Answer from the drawing. Dimensions are ordinates in mm from the lowest x, y and z of the part. A direction names the side the tool comes from. Give positions to 0.01 mm unless a question says otherwise; leave off trailing zeros. Write each loop counter-clockwise with the first axis right and the second up, starting at its lowest first coordinate (ties: lowest second). Pieces come first, ordered by that corner, then holes.
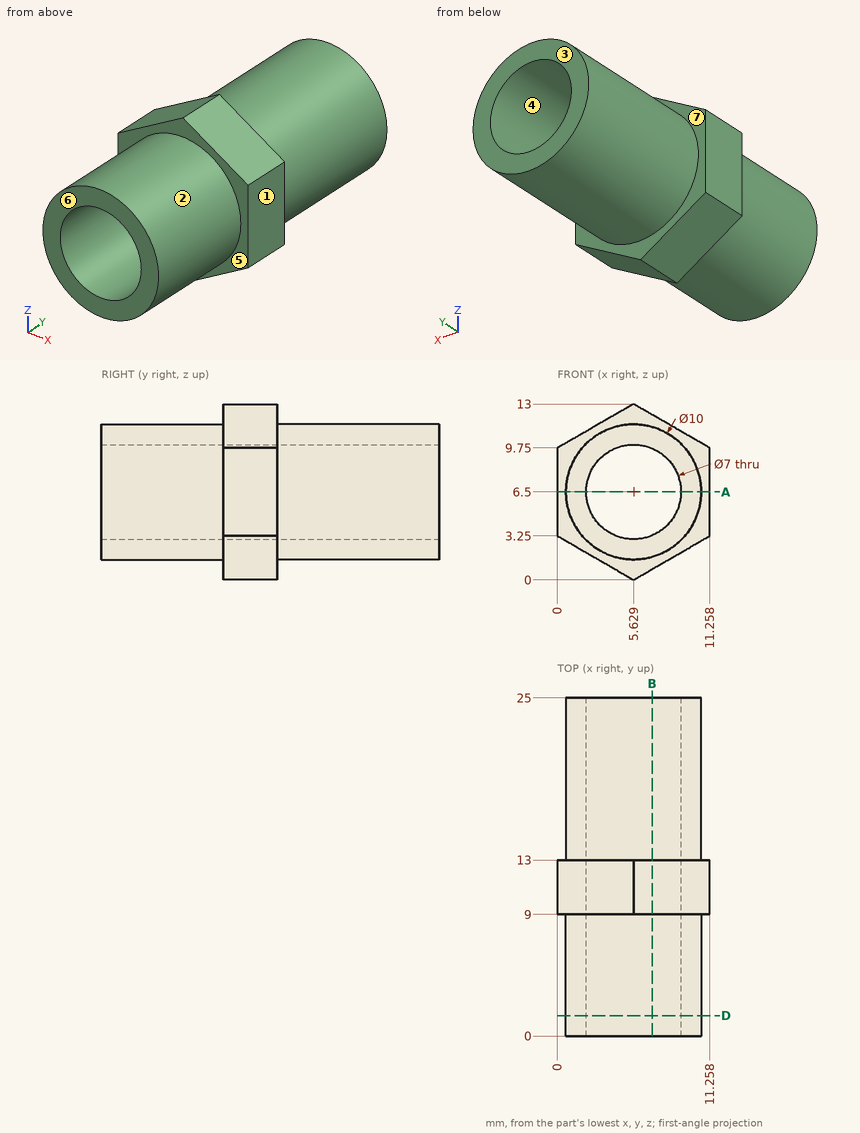
Item 1: A cutting plane is placed at D-D, the plane y = 1.5. Give the vertices of the cut face in (x, z).
Conclusion:
outline: circle Ø10 at (5.63, 6.5); hole circle Ø7 at (5.63, 6.5)
Item 2: Consider probe 1 along Z at (x, y) = (8, 12.5) (1 decimal); probe 2 along X at (y, z) = (18, 3.5) (1 decimal); probe 3 along Z at (x, y) = (4.5, 8.75). Determine where each line is inside the solid, lowest interval first.
Conclusion:
probe 1: z = 1.4 to 3.9, 9.1 to 11.6
probe 2: x = 1.6 to 3.8, 7.4 to 9.6
probe 3: z = 1.63 to 3.19, 9.81 to 11.37
Item 3: A cutting plane is placed at B-B, the plane x = 7. Give the vertices of the cut face in (y, z).
Conclusion:
outline: (0, 1.69) - (9, 1.69) - (9, 0.79) - (13, 0.79) - (13, 1.69) - (25, 1.69) - (25, 3.28) - (0, 3.28) - close; (0, 9.72) - (25, 9.72) - (25, 11.31) - (13, 11.31) - (13, 12.21) - (9, 12.21) - (9, 11.31) - (0, 11.31) - close
Item 4: A cutting plane is placed at A-A, the plane z = 6.5. Give the vertices of the cut face in (x, y).
Conclusion:
outline: (0, 9) - (0.63, 9) - (0.63, 0) - (2.13, 0) - (2.13, 25) - (0.63, 25) - (0.63, 13) - (0, 13) - close; (9.13, 0) - (10.63, 0) - (10.63, 9) - (11.26, 9) - (11.26, 13) - (10.63, 13) - (10.63, 25) - (9.13, 25) - close
Item 5: Which of the six approach directions +Z, -Z, +X, -X, +Y, -Y give full straight-line access (tool end or side, diameter ignored) to the marked faces 5, 6 and 7?
Conclusion:
face 5: -Y
face 6: +Z, -Z, +X, -X, -Y
face 7: +Y
Item 6: Each of these flat-tipped pins is pushed along its axis until it touches: P1, Ø2, axis at x = 8.5, y = 14.5, coming from the +Z side; P2, Ø5, axis at y = 20, z = 2, coming from the +X side; P3, Ø1.5, axis at x = 2.5, y = 10, coming from the -Z side. Where does it stop, or does it pass through?
Conclusion:
P1: stops at z = 11.14
P2: stops at x = 10.21
P3: stops at z = 1.37
Item 7: Determine the mould class of the marked faces 1, 2, 3 and 4 for opening direction X: pulls with the +X half, pulls with the -X half, needs draft (parallel to the pull), parting line crosses it, or undercut.
Conclusion:
face 1: pulls with the +X half
face 2: parting line crosses it
face 3: needs draft
face 4: undercut
